Build history of the part. All positions in model axes, mm. A direction names the side the tool comes from. Coordinates: 2 decimals unless noted, no trailing zeros. Order: outer loops, then holes, each group sorted by start corner. A loop starts at its lowest first (then second) coordinate and runs counter-clockwise, first axis right, second up. Notation, with made-up numbers: (76.5, 71.25) - (107.5, 71.25) arc R21 cw to (107.5, 76.25) - close; hole circle Ø9 at (-15, 69). An arc over 180 degrees is marked (long way). Answer as CSV lines item,"result". Start each with the question number.
from build123d import *

# Parameters (mm, degrees)
SKETCH2_W               = 57.15
SKETCH2_H               = 57.15
BOSS_EXTRUDE2_DEPTH     = 31.75
SKETCH3_R               = 15.875
CUT_EXTRUDE1_DEPTH      = 87.834944003
CUT_EXTRUDE2_DEPTH      = 2.54
FILLET1_R               = 3.175
F_1_4_20_TAPPED_HOLE1_D = 5.1054


with BuildPart() as part:
    # Sketch2 → Boss-Extrude2 (new body)
    with BuildSketch(Plane(origin=(0, 0, 0), x_dir=(0, 0, -1), z_dir=(1, 0, 0))):
        with Locations((28.575, 28.575)):
            Rectangle(SKETCH2_W, SKETCH2_H)
    extrude(amount=BOSS_EXTRUDE2_DEPTH)

    # Sketch3 → Cut-Extrude1 (cut, through all)
    with BuildSketch(Plane(origin=(31.75, 0, 0), x_dir=(0, 0, -1), z_dir=(1, 0, 0))):
        with Locations((28.575, 28.575)):
            Circle(SKETCH3_R)
    extrude(amount=-CUT_EXTRUDE1_DEPTH, mode=Mode.SUBTRACT)

    # Sketch4 → Cut-Extrude2 (cut)
    with BuildSketch(Plane.ZY):
        with BuildLine():
            Line((-36.188382543, 46.0375), (-20.961617457, 46.0375))
            ThreePointArc((-20.961617457, 46.0375), (-9.525, 28.575), (-20.961617457, 11.1125))
            Line((-20.961617457, 11.1125), (-36.188382543, 11.1125))
            ThreePointArc((-36.188382543, 11.1125), (-47.625, 28.575), (-36.188382543, 46.0375))
        make_face()
    extrude(amount=-CUT_EXTRUDE2_DEPTH, mode=Mode.SUBTRACT)

    # Fillet1
    fillet1_edges = [part.edges().sort_by_distance(p)[0] for p in [
        (1.27, 11.1125, -36.188382543),
        (1.27, 46.0375, -36.188382543),
        (1.27, 46.0375, -20.961617457),
        (1.27, 11.1125, -20.961617457),
    ]]
    fillet(fillet1_edges, radius=FILLET1_R)

    # 1/4-20 Tapped Hole1 (through all)
    with Locations(Plane(origin=(31.75, 0, 0), x_dir=(0, 0, -1), z_dir=(1, 0, 0))):
        with Locations((6.35, 50.8), (50.8, 50.8), (50.8, 6.35), (6.35, 6.35), (28.575, 28.575)):
            Hole(F_1_4_20_TAPPED_HOLE1_D / 2)


solid = part.part
(1) Band-saw the part on D-D on y = 26. List the corners of the cut face in (x, z), plus the area to 3 significant figures.
(2) Pull direction Y, two halves, no side cores. Call faces 3 (the flat face through (16, 0, -28)), 4 (the cylindrical face through (15.653, 4.085, -5.172)), 5 (the flat face through (16, 28, 0)), 6 (the flat face through (16, 57.15, -28)): +Y half, -Y half, draft (parallel to the pull), parting line (faces both ways), or undercut.
(3) Which spindle directions (+Z, -Z, +X, -X, +Y, -Y) get a long thin tool onto all of the face, cutting with end or side? Do faces 1 (the cylindrical face through (15.653, 4.085, -49.622)), 2 (the cylindrical face through (1.288, 11.195, -20.936)). Say none if no direction does.
(4) Band-saw the part on B-B on y = 6.35. List the corners of the cut face in (x, z), plus the area to 3 significant figures.
(5) Band-saw the part on A-A on z = -50.8. List the corners of the cut face in (x, y), plus the area to 3 significant figures.
(6) Drop flat-ended pins along their axis: pin 1 Ø4 at (y, z) = (6.35, -6.35) entering from -X; pin 2 Ø3 at (y, z) = (26, -43) entering from -X. Give the stop position or say it passes through.
(7) Probe L1, parallel to Y at x = 16, z = -6.35; L2, parallel to Z at x = 10, y = 4.5; L3, parallel to Z at x = 12, y = 50. List the from-to ranges inside material, lowest first. Write a range as [from, to].
(8) Band-saw the part on C-C on z = -39.5. List the corners of the cut face in (x, y), plus the area to 3 significant figures.
Filled in:
1,outline,"(0, -57.15) - (31.75, -57.15) - (31.75, -44.24) - (2.54, -44.24) - (2.54, -47.45) - (0, -47.45) - close; (0, -9.7) - (2.54, -9.7) - (2.54, -12.91) - (31.75, -12.91) - (31.75, 0) - (0, 0) - close"
1,area,"803 mm^2"
2,face 3,"-Y half"
2,face 4,"undercut"
2,face 5,"draft"
2,face 6,"+Y half"
3,face 1,"+X, -X"
3,face 2,"-X"
4,outline,"(0, -57.15) - (31.75, -57.15) - (31.75, -53.35) - (0, -53.35) - close; (0, -48.25) - (31.75, -48.25) - (31.75, -8.9) - (0, -8.9) - close; (0, -3.8) - (31.75, -3.8) - (31.75, 0) - (0, 0) - close"
4,area,"1,490 mm^2"
5,outline,"(0, 0) - (31.75, 0) - (31.75, 3.8) - (0, 3.8) - close; (0, 8.9) - (31.75, 8.9) - (31.75, 48.25) - (0, 48.25) - close; (0, 53.35) - (31.75, 53.35) - (31.75, 57.15) - (0, 57.15) - close"
5,area,"1,490 mm^2"
6,pin 1,"passes through"
6,pin 2,"stops at x = 2.54"
7,L1,"y = [0, 3.8], [8.9, 48.25], [53.35, 57.15]"
7,L2,"z = [-57.15, -52.56], [-49.04, -8.11], [-4.59, 0]"
7,L3,"z = [-57.15, -53.22], [-48.38, -8.77], [-3.93, 0]"
8,outline,"(0, 0) - (31.75, 0) - (31.75, 17.06) - (2.54, 17.06) - (2.54, 12.97) - (0, 12.97) - close; (0, 44.18) - (2.54, 44.18) - (2.54, 40.09) - (31.75, 40.09) - (31.75, 57.15) - (0, 57.15) - close"
8,area,"1,060 mm^2"
